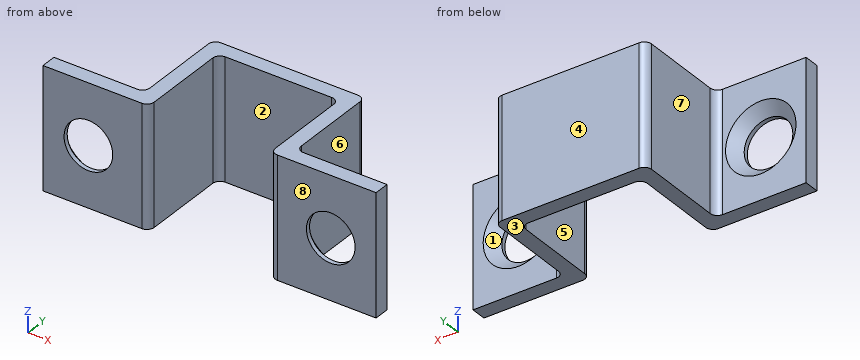
```python
from build123d import *

# Parameters (mm, degrees)
SKETCH1_W           = 12.7
SKETCH1_H           = 12.7
BOSS_EXTRUDE1_DEPTH = 1.6002
SKETCH2_W           = 12.7
SKETCH2_H           = 11.7602
BOSS_EXTRUDE2_DEPTH = 1.6002
SKETCH3_W           = 12.7
SKETCH3_H           = 1.6002
BOSS_EXTRUDE3_DEPTH = 9.525
SKETCH4_R           = 2.5527
CUT_EXTRUDE1_DEPTH  = 22.187985158
FILLET1_R           = 0.762
CHAMFER2_SIZE       = 1.143


with BuildPart() as part:
    # Sketch1 → Boss-Extrude1 (new body)
    with BuildSketch(Plane(origin=(0, 0, 0), x_dir=(1, 0, 0), z_dir=(0, 1, 0))):
        Rectangle(SKETCH1_W, SKETCH1_H)
    extrude(amount=BOSS_EXTRUDE1_DEPTH)

    # Sketch2 → Boss-Extrude2 (add)
    with BuildSketch(Plane(origin=(6.35, 0, 0), x_dir=(0, 0, -1), z_dir=(1, 0, 0))):
        with Locations((0, -4.2799)):
            Rectangle(SKETCH2_W, SKETCH2_H)
    boss_extrude2 = extrude(amount=BOSS_EXTRUDE2_DEPTH)

    # Sketch3 → Boss-Extrude3 (add)
    with BuildSketch(Plane(origin=(7.9502, 0, 0), x_dir=(0, 0, -1), z_dir=(1, 0, 0))):
        with Locations((0, -9.3599)):
            Rectangle(SKETCH3_W, SKETCH3_H)
    boss_extrude3 = extrude(amount=BOSS_EXTRUDE3_DEPTH)

    # Sketch4 → Cut-Extrude1 (cut, through all)
    with BuildSketch(Plane(origin=(0, -8.5598, 0), x_dir=(1, 0, 0), z_dir=(0, 1, 0))):
        with Locations(Location((12.7127, 0, 0), (0, 0, 270))):
            Circle(SKETCH4_R)
    cut_extrude1 = extrude(amount=-CUT_EXTRUDE1_DEPTH, mode=Mode.SUBTRACT)

    # Mirror2: Boss-Extrude2, Boss-Extrude3, Cut-Extrude1 across plane
    add(boss_extrude2.mirror(Plane(origin=(0, 0, 0), x_dir=(0, 0, 1), z_dir=(1, 0, 0))))
    add(boss_extrude3.mirror(Plane(origin=(0, 0, 0), x_dir=(0, 0, 1), z_dir=(1, 0, 0))))
    add(cut_extrude1.mirror(Plane(origin=(0, 0, 0), x_dir=(0, 0, 1), z_dir=(1, 0, 0))), mode=Mode.SUBTRACT)

    # Fillet1
    fillet1_edges = [part.edges().sort_by_distance(p)[0] for p in [
        (6.35, -10.16, 0),
        (-6.35, -10.16, 0),
        (6.35, 0, 0),
        (-6.35, 0, 0),
        (-7.9502, -8.5598, 0),
        (-7.9502, 1.6002, 0),
        (7.9502, 1.6002, 0),
        (7.9502, -8.5598, 0),
    ]]
    fillet(fillet1_edges, radius=FILLET1_R)

    # Chamfer2
    chamfer2_edges = [part.edges().sort_by_distance(p)[0] for p in [
        (12.7127, -8.5598, -2.5527),
        (-12.7127, -8.5598, -2.5527),
    ]]
    chamfer(chamfer2_edges, length=CHAMFER2_SIZE)


solid = part.part
```
Build history of the part. All positions in model axes, mm. Face numbers are marked on the shaded views. A direction names the side the tool comes from. Round coordinates to 2 decimals unless told otherwise and drop trailing zeros. Order: outer loops, then holes, each group sorted by start corner. A loop starts at its lowest first (then second) coordinate and runs counter-clockwise, first axis right, second up. Notation, with made-up numbers: (14.25, -1) -> (28.25, -1) arc R26 ccw to (28.25, 22) -> close; hole circle Ø2 at (19, -32.5). An arc over 180 degrees is marked (long way). Answer in a Markdown table with one row per item.
1) Mould opens along Z. For the marked faces 1, 2 and 3 say: released by +Z, released by -Z, zero draft, split by the parting line, or undercut.
Values:
| item | result |
|---|---|
| face 1 | undercut |
| face 2 | zero draft |
| face 3 | released by -Z |
2) Band-saw the part on B-B on z = 0. Give the number of separate pieces and of enclosed holes in the cut face, and give its area (3 significant figures).
Values:
| item | result |
|---|---|
| separate pieces | 3 |
| enclosed holes | 0 |
| area | 69.5 mm2 |
3) Pin check, flat tips, straight feed: P1, Ø3, axis at y = -1.5, z = -4.5, coming from the +X side; P2, Ø7, axis at x = -14, z = -1.5, coming from the +Y side; P3, Ø4.5, axis at y = -3.5, z = 1.5, coming from the -X side. Stop position of each tip, or through.
Values:
| item | result |
|---|---|
| P1 | x = 7.95 |
| P2 | y = -8.56 |
| P3 | x = -7.95 |
4) Band-saw the part on D-D on x = -3. Give the cut face in (y, z).
Values:
| item | result |
|---|---|
| outline | (0, -6.35) -> (1.6, -6.35) -> (1.6, 6.35) -> (0, 6.35) -> close |
5) Band-saw the part on A-A on y = -3.25. Give the cut face in (x, z).
Values:
| item | result |
|---|---|
| outline | (-7.95, -6.35) -> (-6.35, -6.35) -> (-6.35, 6.35) -> (-7.95, 6.35) -> close; (6.35, -6.35) -> (7.95, -6.35) -> (7.95, 6.35) -> (6.35, 6.35) -> close |
6) Band-saw the part on C-C on z = 4.5. Give the cut face in (x, y), and give its area (3 significant figures).
Values:
| item | result |
|---|---|
| outline | (-17.48, -10.16) -> (-7.11, -10.16) arc R0.76 ccw to (-6.35, -9.4) -> (-6.35, -0.76) arc R0.76 cw to (-5.59, 0) -> (5.59, 0) arc R0.76 cw to (6.35, -0.76) -> (6.35, -9.4) arc R0.76 ccw to (7.11, -10.16) -> (17.48, -10.16) -> (17.48, -8.56) -> (8.71, -8.56) arc R0.76 cw to (7.95, -7.8) -> (7.95, 0.84) arc R0.76 ccw to (7.19, 1.6) -> (-7.19, 1.6) arc R0.76 ccw to (-7.95, 0.84) -> (-7.95, -7.8) arc R0.76 cw to (-8.71, -8.56) -> (-17.48, -8.56) -> close |
| area | 88.4 mm2 |
7) Which spindle directions (+Z, -Z, +X, -X, +Y, -Y) get a long thin tool onto all of the face, cutting with end or side? Do the marked faces 4, 5, 6, 7 and 8. Say none if no direction does.
Values:
| item | result |
|---|---|
| face 4 | +Z, -Z, +X, -X, +Y |
| face 5 | +Z, -Z, -Y |
| face 6 | +Z, -Z, +X, +Y |
| face 7 | +Z, -Z, -X, +Y |
| face 8 | +Z, -Z, +X, -X, -Y |
8) Wall check: L1, parallel to X at y = -1.25, z = -1.25; L2, parallel to X at y = -9.95, z = 0; L3, parallel to Y at x = -0.5, z = -1. Give the ranges that are in metal, low to high.
Values:
| item | result |
|---|---|
| L1 | -7.95 to -6.35, 6.35 to 7.95 |
| L2 | -17.48 to -15.27, -10.16 to -6.59, 6.59 to 10.16, 15.27 to 17.48 |
| L3 | 0 to 1.6 |
